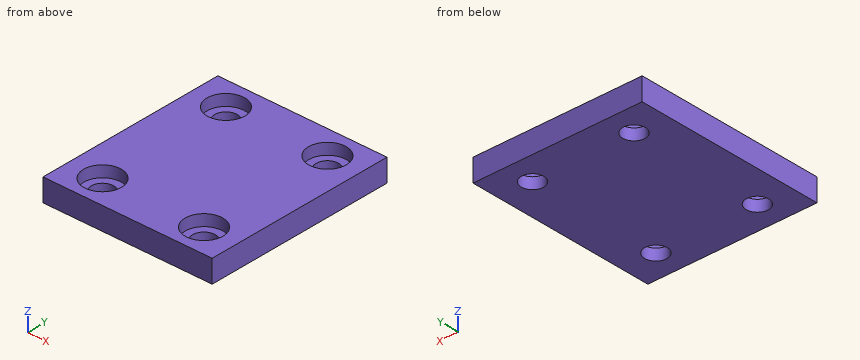
```python
from build123d import *

# Parameters (mm, degrees)
F0_W     = 30
F0_H     = 34
F0_R     = 3.35
F1_DEPTH = 4
F0_R_2   = 2
F2_DEPTH = 2


with BuildPart() as f1:
    # F0 (on Top) → F1 (new body)
    with BuildSketch(Plane.XY):
        with Locations((1.999535, 3.282795)):
            Rectangle(F0_W, F0_H)
        with Locations((-7.000465, -8.717205)):
            Circle(F0_R, mode=Mode.SUBTRACT)
        with Locations((10.999535, -8.717205)):
            Circle(F0_R, mode=Mode.SUBTRACT)
        with Locations((-7.000465, 15.282795)):
            Circle(F0_R, mode=Mode.SUBTRACT)
        with Locations((10.999535, 15.282795)):
            Circle(F0_R, mode=Mode.SUBTRACT)
    extrude(amount=F1_DEPTH)

    # F0 (on Top) → F2 (join)
    with BuildSketch(Plane.XY):
        with Locations((-7.000465, 15.282795)):
            Circle(F0_R)
        with Locations((-7.000465, 15.282795)):
            Circle(F0_R_2, mode=Mode.SUBTRACT)
        with Locations((10.999535, 15.282795)):
            Circle(F0_R)
        with Locations((10.999535, 15.282795)):
            Circle(F0_R_2, mode=Mode.SUBTRACT)
        with Locations((10.999535, -8.717205)):
            Circle(F0_R)
        with Locations((10.999535, -8.717205)):
            Circle(F0_R_2, mode=Mode.SUBTRACT)
        with Locations((-7.000465, -8.717205)):
            Circle(F0_R)
        with Locations((-7.000465, -8.717205)):
            Circle(F0_R_2, mode=Mode.SUBTRACT)
    extrude(amount=F2_DEPTH)


solid = f1.part
```
Read the model definition and answer for the solid it produces. Units are mm, in the model's axes. Coordinates: 2 decimals unless noted, no trailing zeros. Order: outer loops, then holes, each group sorted by start corner. A loop starts at its lowest first (then second) coordinate and runs counter-clockwise, first axis right, second up. Notation, with made-up numbers: (79.25, 6.25) - (120.25, 6.25) arc R29 cw to (120.25, 35.25) - close; hole circle Ø2 at (76, 61.25). An arc over 180 degrees is marked (long way). Answer as a JSON object with one key per item and string values. Group by question number.
Item 1: A flat-ended cylindrical pin translates along its axis: P1, Ø5.5, axis at x = 11, y = 15.28, coming from the +Z side. Find the tip coordinate at first contact, or state that the pin passes through.
Item 2: Consider probe 1 along X at (y, z) = (-7, 0.7); probe 2 along Y at (x, z) = (12.5, 2.45); probe 3 along Z at (x, y) = (14, 14.5). Determine where each line is inside the solid, lowest interval first. Write a range as from..to.
Item 3: Section A-A (y = 16) is taken. Give the vertices of the cut face in (x, z), plus the area to 3 significant figures.
Item 4: Section C-C (z = 0.9) is taken. Give the vertices of the cut face in (x, y).
Item 5: Section D-D (z = 3.3) is taken. Give the vertices of the cut face in (x, y).
Item 6: Section B-B (x = 10) is taken. Give the vertices of the cut face in (y, z).
Results are:
{
 "1": {"P1": "stops at z = 2"},
 "2": {"probe 1": "x = -13..-8.03, -5.98..9.97, 12.02..17", "probe 2": "y = -13.72..-11.71, -5.72..12.29, 18.28..20.28", "probe 3": "z = 0..2"},
 "3": {"outline": "(-13, 0) - (-8.87, 0) - (-8.87, 2) - (-10.27, 2) - (-10.27, 4) - (-13, 4) - close; (-5.13, 0) - (9.13, 0) - (9.13, 2) - (7.73, 2) - (7.73, 4) - (-3.73, 4) - (-3.73, 2) - (-5.13, 2) - close; (12.87, 0) - (17, 0) - (17, 4) - (14.27, 4) - (14.27, 2) - (12.87, 2) - close", "area": "78.9 mm^2"},
 "4": {"outline": "(-13, -13.72) - (17, -13.72) - (17, 20.28) - (-13, 20.28) - close; hole circle Ø4 at (-7, -8.72); hole circle Ø4 at (-7, 15.28); hole circle Ø4 at (11, -8.72); hole circle Ø4 at (11, 15.28)"},
 "5": {"outline": "(-13, -13.72) - (17, -13.72) - (17, 20.28) - (-13, 20.28) - close; hole circle Ø6.7 at (-7, -8.72); hole circle Ø6.7 at (-7, 15.28); hole circle Ø6.7 at (11, -8.72); hole circle Ø6.7 at (11, 15.28)"},
 "6": {"outline": "(-13.72, 0) - (-10.45, 0) - (-10.45, 2) - (-11.91, 2) - (-11.91, 4) - (-13.72, 4) - close; (-6.98, 0) - (13.55, 0) - (13.55, 2) - (12.09, 2) - (12.09, 4) - (-5.52, 4) - (-5.52, 2) - (-6.98, 2) - close; (17.02, 0) - (20.28, 0) - (20.28, 4) - (18.48, 4) - (18.48, 2) - (17.02, 2) - close"}
}
